Could you check a few things on this model? Use its own coordinates, in mm. A direction names the side the tool comes from. Coordinates: 2 decimals unless noted, no trailing zeros. Write each loop counter-clockwise with the first axis right and the second up, starting at its lowest first coordinate (ties: lowest second). Pieces come first, ordered by that corner, then holes. Notation, with made-up numbers: M 38,-15 L 72,-15 A17 ccw 72,-10 Z; hole C -15,60.25 d4. An arc over 180 degrees is marked long. Answer as CSV lines item,"result". Start each with the question number.
Item 1: We'd pull the mould along Y, two halves only. Please class faces 1 (the flat face through (0, 128, 9)), 2 (the cylindrical face through (161.193, 252.793, 16.334)), 3 (the cylindrical face through (160.54, 19.16, 8.31)): +Y half, -Y half, draft (parallel to the pull), parting line (faces both ways), or undercut.
Item 2: Suppose I cut it at C-C, the plane y = 218. Write out the boundary of the cut face in (x, z), and give its area (3 significant figures).
Item 3: On a 3-axis mill with a long thin cutter (end or side, diameter ignored), from which of +Z, -Z, +X, -X, +Y, -Y can I reach the whole of each face in a straight line? I mean faces 4 (the cylindrical face through (161.2, 1.23, 16.33)), 5 (the flat face through (19.05, 126, 9)), 6 (the flat face through (1.473, 128, 9)). Say none if no direction works.
Item 4: If I drill on line 1 along X through (y, z) = (165, 14.5); line 2 along Y through (x, z) = (36, 10.5); line 3 along Y through (x, z) = (125, 7), over which ranges is the centre line in solid material (lowest first)? Write a range as [from, to].
Item 5: I'm going to push flat-ended pins straight in: P1, Ø5, axis at y = 113.5, z = 7.5, coming from the +X side; P2, Ø5, axis at x = 76.5, z = 2, coming from the -Y side; P3, Ø4, axis at x = 23, z = 6.5, coming from the -Y side. Where does each tip first touch, or does it pass through?
Item 6: Suppose I cut it at A-A, the plane y = 76.5. Write out the boundary of the cut face in (x, z), and give its area (3 significant figures).
Item 7: Suppose I cut it at B-B, the plane x = 132.5. Write out the boundary of the cut face in (y, z), and give its area (3 significant figures).
```python
from build123d import *

# Parameters (mm, degrees)
F1_DEPTH  = 19.05
F2_T      = -1.4732
F3_W      = 16.1036
F3_H      = 19.05
F4_DEPTH  = 25.4
F5_R      = 9.52499
F6_R      = 3.175
F7_DEPTH  = 250.7881261572
F8_W      = 16.1036
F8_H      = 19.05
F9_DEPTH  = 25.4
F10_R     = 9.52499
F11_R     = 3.175
F12_DEPTH = 250.7881261572


# Not quite as in the source:
# - a fillet or chamfer is up to 0.001 mm smaller than in the source, because OpenCascade refuses the exact size


with BuildPart() as f1:
    # F0 (on Top) → F1 (new body)
    with BuildSketch(Plane.XY):
        Polygon((0, 225.425), (0, 28.575), (163.8898551464, 0), (167.1619531291, 18.766882394), (19.05, 44.5909277987), (19.05, 209.4090722013), (167.1619531291, 235.233117606), (163.8898551464, 254), align=None)
    extrude(amount=F1_DEPTH)

    # F2
    f2_openings = [f1.faces().sort_by_distance(p)[0] for p in [
        (165.525904, 9.383441, 9.525),
        (165.525904, 244.616559, 9.525),
    ]]
    offset(amount=F2_T, openings=f2_openings, kind=Kind.INTERSECTION)

    # F3 (on face) → F4 (cut)
    with BuildSketch(Plane(origin=(159.0546521525, -27.731958645, 0), x_dir=(0.1717636736, 0.9851381834, 0), z_dir=(0.9851381834, -0.1717636736, 0))):
        with Locations((37.6753235911, 9.525)):
            Rectangle(F3_W, F3_H)
    extrude(amount=-F4_DEPTH, mode=Mode.SUBTRACT)

    # F5 (radius 9.525 in the source; OpenCascade refuses exactly that, so slightly less here)
    f5_edges = [f1.edges().sort_by_distance(p)[0] for p in [
        (164.016376, 0.725653, 19.05),
        (167.035432, 18.04123, 19.05),
        (164.016376, 0.725653, 0),
        (167.035432, 18.04123, 0),
    ]]
    fillet(f5_edges, radius=F5_R)

    # F6 (on face) → F7 (cut, through all)
    with BuildSketch(Plane(origin=(4.8352029939, 27.731958645, 0), x_dir=(0.9851381834, -0.1717636736, 0), z_dir=(-0.1717636736, -0.9851381834, 0))):
        with Locations((151.9291541789, 9.525)):
            Circle(F6_R)
    extrude(amount=-F7_DEPTH, mode=Mode.SUBTRACT)

    # F8 (on face) → F9 (cut)
    with BuildSketch(Plane(origin=(202.0342343209, 35.2256595783, 0), x_dir=(-0.1717636736, 0.9851381834, 0), z_dir=(0.9851381834, 0.1717636736, 0))):
        with Locations((212.5497749961, 9.525)):
            Rectangle(F8_W, F8_H)
    extrude(amount=-F9_DEPTH, mode=Mode.SUBTRACT)

    # F10 (radius 9.525 in the source; OpenCascade refuses exactly that, so slightly less here)
    f10_edges = [f1.edges().sort_by_distance(p)[0] for p in [
        (164.016376, 253.274347, 0),
        (164.016376, 253.274347, 19.05),
        (167.035432, 235.95877, 19.05),
        (167.035432, 235.95877, 0),
    ]]
    fillet(f10_edges, radius=F10_R)

    # F11 (on face) → F12 (cut, through all)
    with BuildSketch(Plane(origin=(-38.1443791745, 218.7743404217, 0), x_dir=(-0.9851381834, -0.1717636736, 0), z_dir=(-0.1717636736, 0.9851381834, 0))):
        with Locations((-195.5571272816, 9.525)):
            Circle(F11_R)
    extrude(amount=-F12_DEPTH, mode=Mode.SUBTRACT)


solid = f1.part
```
Ans:
1,face 1,"draft"
1,face 2,"+Y half"
1,face 3,"undercut"
2,outline,"M 0,0 L 68.32,0 L 68.32,19.05 L 0,19.05 Z; hole M 1.47,1.47 L 59.75,1.47 L 59.75,17.58 L 1.47,17.58 Z"
2,area,"363 mm^2"
3,face 4,"+Z, +X, -Y"
3,face 5,"+Z, -Z, +X"
3,face 6,"none"
4,line 1,"x = [0, 1.47], [17.58, 19.05]"
4,line 2,"y = [22.3, 23.79], [40.14, 41.64], [212.36, 213.86], [230.21, 231.7]"
4,line 3,"y = [6.78, 8.28], [24.62, 26.12], [227.88, 229.38], [245.72, 247.22]"
5,P1,"stops at x = 19.05"
5,P2,"stops at y = 14.8"
5,P3,"stops at y = 24.22"
6,outline,"M 0,0 L 19.05,0 L 19.05,19.05 L 0,19.05 Z; hole M 1.47,1.47 L 17.58,1.47 L 17.58,17.58 L 1.47,17.58 Z"
6,area,"104 mm^2"
7,outline,"M 5.47,0 L 24.81,0 L 24.81,19.05 L 5.47,19.05 Z; M 229.19,0 L 248.53,0 L 248.53,19.05 L 229.19,19.05 Z; hole M 6.97,1.47 L 23.31,1.47 L 23.31,17.58 L 6.97,17.58 Z; hole M 230.69,1.47 L 247.03,1.47 L 247.03,17.58 L 230.69,17.58 Z"
7,area,"210 mm^2"
